Read the model definition and answer for the solid it produces. Units are mm, in the model's axes. A direction names the side the tool comes from. Give positions to 0.01 mm unless a question says otherwise; leave off trailing zeros. Loops run counter-clockwise (first coordinate to the right, second up) from the corner with the lowest first, then second, coordinate; pieces in that order, holes last. Notation, with made-up numbers: (17.5, 48.5) - (24.5, 48.5) arc R29 ccw to (24.5, 76.5) - close; hole circle Ø10 at (-2, 14.5). An arc over 180 degrees is marked (long way). Write item = value, one per line. Start each with the question number.
from build123d import *

# Parameters (mm, degrees)
F4_SIZE       = 1
F5_W          = 43
F5_H          = 3
F6_DEPTH      = 21.001
F6_DEPTH_BACK = 21.001
F7_R          = 7
F8_DEPTH      = 71.001


with BuildPart() as f1:
    # F0 (on Front) → F1 (revolve)
    with BuildSketch(Plane.XZ):
        Polygon((43, 15), (43, 21), (0, 21), (0, 11), (2.5, 11), (2.5, 12.5), (17.5, 12.5), (17.5, 15), align=None)
    revolve(axis=Axis((10.041691, 0, 0), (1, 0, 0)))

    # F4
    f4_edges = [f1.edges().sort_by_distance(p)[0] for p in [
        (43, 0, -15),
        (17.5, 0, -12.5),
    ]]
    chamfer(f4_edges, length=F4_SIZE)

    # F5 (on Front) → F6 (cut, two sides)
    with BuildSketch(Plane.XZ) as f6_sk:
        with Locations((21.5, 20.5)):
            Rectangle(F5_W, F5_H)
        with Locations((21.5, -20.5)):
            Rectangle(F5_W, F5_H)
    extrude(amount=F6_DEPTH, mode=Mode.SUBTRACT)
    extrude(f6_sk.sketch, amount=-F6_DEPTH_BACK, mode=Mode.SUBTRACT)

    # F7 (on offset) → F8 (cut, through all)
    with BuildSketch(Plane.XZ.offset(50)):
        with Locations((33, 21.99)):
            Circle(F7_R)
    extrude(amount=-F8_DEPTH, mode=Mode.SUBTRACT)


solid = f1.part
1. A cutting plane is placed at A-A on z = 0. Give the vertices of the cut face in (x, y).
2. A cutting plane is placed at D-D on x = 35.5. Give the vertices of the cut face in (y, z), and give its area (3 significant figures).
3. A tool of negligible diameter and unlimited length cuts with its end or side. For faces 1 (the cylindrical face through (21, 21, 0)), 2 (the flat face through (17.5, -7.85, 11.18)), from which of +Z, -Z, +X, -X, +Y, -Y can it reach the whole face along a straight path? Write none if from no direction.
4. For a pull along Y with two mould halves and no side action, classify faces 3 (the flat face through (2.5, 10, -5)), 4 (the cylindrical face through (21, -21, 0)), 5 (the flat face through (43, 13.9, -8.4)) as released by +Y, released by -Y, zero draft, split by the parting line, or undercut.
5. A cutting plane is placed at B-B on y = 0. Give the vertices of the cut face in (x, z).
6. Consider line 1 along Y through (x, z) = (35.25, 0); line 2 along Z through (x, y) = (1.5, 0); line 3 along Z through (x, y) = (22, 0). Determine where each line is inside the solid, lowest interval first. Write a range as [from, to].
7. A cutting plane is placed at C-C on x = 24. Give the vertices of the cut face in (y, z).
8. Given P1, Ø12, axis at y = 0.5, z = 13, coming from the +X side; P2, Ø12, axis at x = 9, z = 15, coming from the -Y side; P3, Ø3, axis at x = 21.5, z = 9, coming from the -Y side; P4, Ø15, axis at y = -5, z = 1.5, coming from the +X side, each flat-ended and moving along its own axis, determine where each tip first touches the part or whether it passes through.
Reply:
q1.outline = (0, -21) - (43, -21) - (43, -16) - (42, -15) - (17.5, -15) - (17.5, -13.5) - (16.5, -12.5) - (2.5, -12.5) - (2.5, -11) - (0, -11) - close; (0, 11) - (2.5, 11) - (2.5, 12.5) - (16.5, 12.5) - (17.5, 13.5) - (17.5, 15) - (42, 15) - (43, 16) - (43, 21) - (0, 21) - close
q2.outline = (-14.22, 15.45) arc R21 ccw to (-8.94, -19) - (8.94, -19) arc R21 ccw to (14.22, 15.45) - close; hole circle Ø30 at (0, 0)
q2.area = 546 mm^2
q3.face_1 = +X, -X, +Y
q3.face_2 = +X
q4.face_3 = undercut
q4.face_4 = released by -Y
q4.face_5 = zero draft
q5.outline = (0, -19) - (43, -19) - (43, -16) - (42, -15) - (17.5, -15) - (17.5, -13.5) - (16.5, -12.5) - (2.5, -12.5) - (2.5, -11) - (0, -11) - close; (0, 11) - (2.5, 11) - (2.5, 12.5) - (16.5, 12.5) - (17.5, 13.5) - (17.5, 15) - (32.63, 15) arc R7 cw to (26.67, 19) - (0, 19) - close; (33.37, 15) - (42, 15) - (43, 16) - (43, 19) - (39.33, 19) arc R7 cw to start
q6.line_1 = [-21, -15], [15, 21]
q6.line_2 = [-19, -11], [11, 19]
q6.line_3 = [-19, -15], [15, 19]
q7.outline = (-8.94, -19) - (8.94, -19) arc R21 ccw to (8.94, 19) - (-8.94, 19) arc R21 ccw to start; hole circle Ø30 at (0, 0)
q8.P1 = 43
q8.P2 = -18.97
q8.P3 = -19.62
q8.P4 = 16.72
